from build123d import *

# Parameters (mm, degrees)
SKETCH_1_W          = 79
SKETCH_1_H          = 32
SKETCH_1_R          = 1.55
EXTRUDE_1_DEPTH     = 5
FILLET_1_R          = 4
SKETCH_2_W          = 63
SKETCH_2_H          = 22
CUT_EXTRUDE_1_DEPTH = 6
FILLET_2_R          = 4


with BuildPart() as part:
    # 草图1 → 凸台-拉伸1 (new body)
    with BuildSketch(Plane(origin=(0, 0, 0), x_dir=(1, 0, 0), z_dir=(0, 1, 0))):
        Rectangle(SKETCH_1_W, SKETCH_1_H)
        with Locations((-37.5, 11)):
            Circle(SKETCH_1_R, mode=Mode.SUBTRACT)
        with Locations((-37.5, -11)):
            Circle(SKETCH_1_R, mode=Mode.SUBTRACT)
        with Locations((37.5, 11)):
            Circle(SKETCH_1_R, mode=Mode.SUBTRACT)
        with Locations((37.5, -11)):
            Circle(SKETCH_1_R, mode=Mode.SUBTRACT)
    extrude(amount=EXTRUDE_1_DEPTH)

    # 圆角1
    fillet_1_edges = [part.edges().sort_by_distance(p)[0] for p in [
        (39.5, 2.5, 16),
        (-39.5, 2.5, 16),
        (-39.5, 2.5, -16),
        (39.5, 2.5, -16),
    ]]
    fillet(fillet_1_edges, radius=FILLET_1_R)

    # 草图2 → 切除-拉伸1 (cut, through all)
    with BuildSketch(Plane(origin=(0, 5, 0), x_dir=(1, 0, 0), z_dir=(0, 1, 0))):
        Rectangle(SKETCH_2_W, SKETCH_2_H)
    extrude(amount=-CUT_EXTRUDE_1_DEPTH, mode=Mode.SUBTRACT)

    # 圆角2
    fillet_2_edges = [part.edges().sort_by_distance(p)[0] for p in [
        (31.5, 2.5, -11),
        (31.5, 2.5, 11),
        (-31.5, 2.5, 11),
        (-31.5, 2.5, -11),
    ]]
    fillet(fillet_2_edges, radius=FILLET_2_R)


solid = part.part
Geometry: final body of the model. Coordinates: model frame, mm. A direction names the side the tool comes from. Give positions to 0.01 mm unless a question says otherwise; leave off trailing zeros. Write each loop counter-clockwise with the first axis right and the second up, starting at its lowest first coordinate (ties: lowest second). Pieces come first, ordered by that corner, then holes. Notation, with made-up numbers: (79.5, -1.75) - (138.5, -1.75) arc R32 ccw to (138.5, 32.25) - close; hole circle Ø3 at (26, 37.25). An arc over 180 degrees is marked (long way). Return JSON: item names as keys, results as strings. Group by question number.
1) Section C-C on z = 4. Return the cut outline in (x, y).
2) Section A-A on x = -9. Return the cut outline in (y, z).
3) Line query: line 1 (Z direction, x = 26, y = 2.5); line 2 (X direction, y = 1.4, z = -3.5); line 3 (Z direction, x = -37.5, y = 1.6). Output: solid intervals per line, ascending.
4) Set-up query: faces 5 (the flat face through (-1, 0, 14)), 6 (the flat face through (-31.5, 3, 0)). Return all of +Z, -Z, +X, -X, +Y, -Y with unobstructed straight access to the full face (end or side cutting, diameter ignored); none if empty.
5) Section D-D on x = 37.5. Return the cut outline in (y, z), plus the area to 3 significant figures.
6) Mould query, pull axis X, two halves, no side actions, for faces 1 (the cylindrical face through (-30.297, 2.465, 9.859)), 2 (the cylindrical face through (-38.359, 2.535, 14.797)), 3 (the flat face through (0, 2, -16)), 4 (the cylindrical face through (38.297, 2.535, 14.859)). Classes: released by +X, released by -X, zero draft, split by the parting line, or undercut.
7) Section B-B on y = 2.7. Return the cut outline in (x, z), plus the area to 3 significant figures.
Filled in:
{
 "1": {"outline": "(-39.5, 0) - (-31.5, 0) - (-31.5, 5) - (-39.5, 5) - close; (31.5, 0) - (39.5, 0) - (39.5, 5) - (31.5, 5) - close"},
 "2": {"outline": "(0, -16) - (5, -16) - (5, -11) - (0, -11) - close; (0, 11) - (5, 11) - (5, 16) - (0, 16) - close"},
 "3": {"line 1": "z = -16 to -11, 11 to 16", "line 2": "x = -39.5 to -31.5, 31.5 to 39.5", "line 3": "z = -15.46 to -12.55, -9.45 to 9.45, 12.55 to 15.46"},
 "4": {"face 5": "+Z, -Z, +X, -X, -Y", "face 6": "+Y, -Y"},
 "5": {"outline": "(0, -15.46) - (5, -15.46) - (5, -12.55) - (0, -12.55) - close; (0, -9.45) - (5, -9.45) - (5, 9.45) - (0, 9.45) - close; (0, 12.55) - (5, 12.55) - (5, 15.46) - (0, 15.46) - close", "area": "124 mm^2"},
 "6": {"face 1": "undercut", "face 2": "released by -X", "face 3": "zero draft", "face 4": "released by +X"},
 "7": {"outline": "(-39.5, -12) arc R4 ccw to (-35.5, -16) - (35.5, -16) arc R4 ccw to (39.5, -12) - (39.5, 12) arc R4 ccw to (35.5, 16) - (-35.5, 16) arc R4 ccw to (-39.5, 12) - close; hole circle Ø3.1 at (-37.5, -11); hole circle Ø3.1 at (-37.5, 11); hole (-31.5, -7) arc R4 ccw to (-27.5, -11) - (27.5, -11) arc R4 ccw to (31.5, -7) - (31.5, 7) arc R4 ccw to (27.5, 11) - (-27.5, 11) arc R4 ccw to (-31.5, 7) - close; hole circle Ø3.1 at (37.5, -11); hole circle Ø3.1 at (37.5, 11)", "area": "1,110 mm^2"}
}
